Work out the finished part from the listing and answer in its coordinate system (mm). A direction names the side the tool comes from. Round coordinates to 2 decimals unless told otherwise and drop trailing zeros. Write each loop counter-clockwise with the first axis right and the second up, starting at its lowest first coordinate (ties: lowest second). Pieces come first, ordered by that corner, then holes.
from build123d import *

# Parameters (mm, degrees)
BOSS_EXTRUDE1_DEPTH = 13
SKETCH2_W           = 5
SKETCH2_H           = 16


with BuildPart() as part:
    # Sketch1 → Boss-Extrude1 (new, symmetric)
    with BuildSketch(Plane(origin=(0, 0, 0), x_dir=(1, 0, 0), z_dir=(0, 1, 0))):
        with BuildLine():
            Line((-59.191435728, -3.155996626), (-79.191435728, -3.155996626))
            ThreePointArc((-79.191435728, -3.155996626), (10.808564272, -93.155996626), (100.808564272, -3.155996626))
            Line((100.808564272, -3.155996626), (80.808564272, -3.155996626))
            ThreePointArc((80.808564272, -3.155996626), (10.808564272, -73.155996626), (-59.191435728, -3.155996626))
        make_face()
    extrude(amount=BOSS_EXTRUDE1_DEPTH, both=True)

    # Sketch2 → Cut-Revolve1 (revolve, cut)
    with BuildSketch(Plane(origin=(0, 0, 3.155996626), x_dir=(-1, 0, 0), z_dir=(0, 0, -1))):
        with Locations((61.691435728, 0)):
            Rectangle(SKETCH2_W, SKETCH2_H)
    revolve(axis=Axis((10.808564272, 13, 3.155996626), (0, -1, 0)), mode=Mode.SUBTRACT)


solid = part.part
Q1. Find the intervals of material crossed by L1, parallel to X at y = 7, z = 27; L2, parallel to X at y = 9.25, z = 44; L3, parallel to Z at x = 9.5, y = -4.5, in increasing order.
Q2. The mould has two halves that part along Y. Classify faces 3 (the face through (12.458, 0.112, 78.138)), 4 (the face through (10, -13, 75)), 5 (the face through (12.35, -10.46, 73.14)), 6 (the face through (10, 13, 75)): +Y half, -Y half, draft (parallel to the pull), parting line (faces both ways), or undercut.
Q3. Find section C-C (y = -6.25). Determine the outline of the cut face in (x, z).
Q4. Find section A-A (z = 57). Determine the outline of the cut face in (x, y), plus the area to 3 significant figures.
Q5. Find section B-B (x = 40.5). Determine the outline of the cut face in (y, z).
Q6. Given pin 1 (5 mm diameter, centred on y = -4.5, z = 75, fed in from -X); pin 2 (6 mm diameter, centred on y = -4, z = 40, fed in from -X); pin 3 (5 mm diameter, centred on y = 1, z = 69.5, fed in from +X), each flat-ended and moving along its own axis, determine where each tip first touches the part or whether it passes through.
Q7. Find section D-D (z = 12). Determine the outline of the cut face in (x, y), plus the area to 3 significant figures.
Q8. A tool of negligible diameter and unlimited length cuts with its end or side. For faces 1 (the face through (-69, 0, 3.156)), 2 (the face through (10, -8, 74)), from which of +Z, -Z, +X, -X, +Y, -Y can it reach the whole face along a straight path? Write none if from no direction.
Report:
1. L1: x = -75.98 to -60.3, 81.92 to 97.59
1. L2: x = -69.39 to -46.04, 67.66 to 91.01
1. L3: z = 78.14 to 93.15
2. face 3: undercut
2. face 4: -Y half
2. face 5: draft
2. face 6: +Y half
3. outline: (-79.19, 3.16) - (-64.19, 3.16) arc R75 cw to (85.81, 3.16) - (100.81, 3.16) arc R90 ccw to start
4. outline: (-61.31, -13) - (-33.92, -13) - (-33.92, -8) - (-41.4, -8) - (-41.4, 8) - (-33.92, 8) - (-33.92, 13) - (-61.31, 13) - close; (55.54, -13) - (82.93, -13) - (82.93, 13) - (55.54, 13) - (55.54, 8) - (63.02, 8) - (63.02, -8) - (55.54, -8) - close
4. area: 1,180 mm2
5. outline: (-13, 66.55) - (-8, 66.55) - (-8, 72.03) - (8, 72.03) - (8, 66.55) - (13, 66.55) - (13, 88.12) - (-13, 88.12) - close
6. pin 1: stops at x = -46.56
6. pin 2: stops at x = -72.59
6. pin 3: stops at x = 74.24
7. outline: (-78.76, -13) - (-58.63, -13) - (-58.63, -8) - (-63.67, -8) - (-63.67, 8) - (-58.63, 8) - (-58.63, 13) - (-78.76, 13) - close; (80.25, -13) - (100.37, -13) - (100.37, 13) - (80.25, 13) - (80.25, 8) - (85.29, 8) - (85.29, -8) - (80.25, -8) - close
7. area: 885 mm2
8. face 1: -Z, +X, -X, +Y, -Y
8. face 2: -Z
